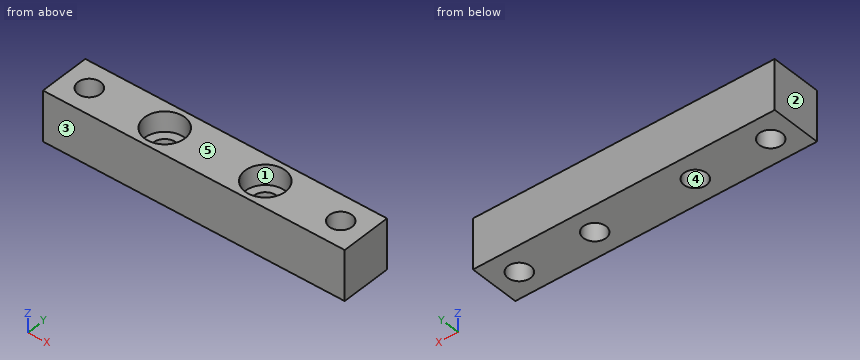
```python
from build123d import *

# Parameters (mm, degrees)
CROQUIS1_W              = 60
CROQUIS1_H              = 10
CROQUIS1_R              = 2.25
SALIENTE_EXTRUIR1_DEPTH = 5
CROQUIS4_R              = 4
CORTAR_EXTRUIR1_DEPTH   = 4


with BuildPart() as part:
    # Croquis1 → Saliente-Extruir1 (new, symmetric)
    with BuildSketch(Plane.XY):
        Rectangle(CROQUIS1_W, CROQUIS1_H)
        with Locations((-10, 0)):
            Circle(CROQUIS1_R, mode=Mode.SUBTRACT)
        with Locations((10, 0)):
            Circle(CROQUIS1_R, mode=Mode.SUBTRACT)
        with Locations((-25, 0)):
            Circle(CROQUIS1_R, mode=Mode.SUBTRACT)
        with Locations(Location((25, 0, 0), (0, 0, 180))):
            Circle(CROQUIS1_R, mode=Mode.SUBTRACT)
    extrude(amount=SALIENTE_EXTRUIR1_DEPTH, both=True)

    # Croquis4 → Cortar-Extruir1 (cut)
    with BuildSketch(Plane.XY.offset(5)):
        with Locations((-10, 0)):
            Circle(CROQUIS4_R)
        with Locations((10, 0)):
            Circle(CROQUIS4_R)
    extrude(amount=-CORTAR_EXTRUIR1_DEPTH, mode=Mode.SUBTRACT)


solid = part.part
```
Work out the finished part from the listing and answer in its coordinate system (mm). Face numbers are marked on the shaded views. A direction names the side the tool comes from. Coordinates: 2 decimals unless noted, no trailing zeros. Loops run counter-clockwise (first coordinate to the right, second up) from the corner with the lowest first, then second, coordinate; pieces in that order, holes last. Notation, with made-up numbers: (45.5, -33) -> (61.5, -33) arc R17 cw to (61.5, -29) -> close; hole circle Ø11 at (84.5, -20). An arc over 180 degrees is marked (long way). Answer as CSV lines item,"result".
Q1. For a pull along Y with two mould halves and no side action, classify the marked faces 3, 4 and 5 as +Y half, -Y half, draft (parallel to the pull), parting line (faces both ways), or undercut.
Findings:
face 3,"-Y half"
face 4,"undercut"
face 5,"draft"
Q2. The part is cut by section C-C on z = -2. Write down the section's boundary in (x, y).
Findings:
outline,"(-30, -5) -> (30, -5) -> (30, 5) -> (-30, 5) -> close; hole circle Ø4.5 at (-25, 0); hole circle Ø4.5 at (-10, 0); hole circle Ø4.5 at (10, 0); hole circle Ø4.5 at (25, 0)"
Q3. Each of these flat-tipped pins is pushed along its axis until it touches: pin 1 (2.5 mm diameter, centred on x = 25, y = 0, fed in from +Z); pin 2 (6 mm diameter, centred on x = -10, y = 0, fed in from +Z). Where does it stop, or does it pass through?
Findings:
pin 1,"passes through"
pin 2,"stops at z = 1"
Q4. A tool of negligible diameter and unlimited length cuts with its end or side. For the marked faces 1 and 2, from which of +Z, -Z, +X, -X, +Y, -Y can it reach the whole face along a straight path? Write none if from no direction.
Findings:
face 1,"+Z"
face 2,"+Z, -Z, -X, +Y, -Y"
Q5. Find the intervals of material crossed by probe 1 along X at (y, z) = (-1.25, -2.75); probe 2 along Y at (x, z) = (-10, -3.45); probe 3 along Y at (x, z) = (10, 2.5), in increasing order.
Findings:
probe 1,"x = -30 to -26.87, -23.13 to -11.87, -8.13 to 8.13, 11.87 to 23.13, 26.87 to 30"
probe 2,"y = -5 to -2.25, 2.25 to 5"
probe 3,"y = -5 to -4, 4 to 5"
Q6. The part is cut by section D-D on y = -3.5. Write down the section's boundary in (x, z), and give its area (3 significant figures).
Findings:
outline,"(-30, -5) -> (30, -5) -> (30, 5) -> (11.94, 5) -> (11.94, 1) -> (8.06, 1) -> (8.06, 5) -> (-8.06, 5) -> (-8.06, 1) -> (-11.94, 1) -> (-11.94, 5) -> (-30, 5) -> close"
area,"569 mm²"
Q7. The part is cut by section A-A on x = -10. Write down the section's boundary in (y, z), and give its area (3 significant figures).
Findings:
outline,"(-5, -5) -> (-2.25, -5) -> (-2.25, 1) -> (-4, 1) -> (-4, 5) -> (-5, 5) -> close; (2.25, -5) -> (5, -5) -> (5, 5) -> (4, 5) -> (4, 1) -> (2.25, 1) -> close"
area,"41.0 mm²"
Q8. The part is cut by section B-B on y = 0. Write down the section's boundary in (x, z), and give its area (3 significant figures).
Findings:
outline,"(-30, -5) -> (-27.25, -5) -> (-27.25, 5) -> (-30, 5) -> close; (-22.75, -5) -> (-12.25, -5) -> (-12.25, 1) -> (-14, 1) -> (-14, 5) -> (-22.75, 5) -> close; (-7.75, -5) -> (7.75, -5) -> (7.75, 1) -> (6, 1) -> (6, 5) -> (-6, 5) -> (-6, 1) -> (-7.75, 1) -> close; (12.25, -5) -> (22.75, -5) -> (22.75, 5) -> (14, 5) -> (14, 1) -> (12.25, 1) -> close; (27.25, -5) -> (30, -5) -> (30, 5) -> (27.25, 5) -> close"
area,"392 mm²"
